Here's how the part is built. I have some questions about the finished solid (model axes, mm). A direction names the side the tool comes from. Round coordinates to 2 decimals unless told otherwise and drop trailing zeros. Order: outer loops, then holes, each group sorted by start corner. A loop starts at its lowest first (then second) coordinate and runs counter-clockwise, first axis right, second up. Notation, with made-up numbers: (50, 75) -> (72, 75) arc R32 cw to (72, 104) -> close; hole circle Ø1 at (-7, 5.25). An arc over 180 degrees is marked (long way). One line per item, written item: value.
```python
from build123d import *

# Parameters (mm, degrees)
BOSS_EXTRUDE1_DEPTH = 40
SKETCH16_R          = 17.5
BOSS_EXTRUDE2_DEPTH = 3
SKETCH17_R          = 16.65
SKETCH17_R_2        = 15.5
BOSS_EXTRUDE3_DEPTH = 10
SKETCH18_R          = 8.5
CUT_EXTRUDE1_DEPTH  = 30
BOSS_EXTRUDE4_DEPTH = 3
FILLET1_R           = 1
FILLET3_R           = 1
BOSS_EXTRUDE5_START = 2
BOSS_EXTRUDE5_DEPTH = 2
CUT_EXTRUDE3_START  = -2
CUT_EXTRUDE3_DEPTH  = 2
SKETCH28_R          = 5.051145337
CUT_EXTRUDE4_DEPTH  = 10


# Read off the part's stored shape, not the designer's step: Cut-Extrude3
with BuildPart() as part:
    # Sketch13 → Boss-Extrude1 (new body)
    with BuildSketch(Plane(origin=(0, 0, 0), x_dir=(1, 0, 0), z_dir=(0, 1, 0))):
        with BuildLine():
            Line((0.65523527, 15.486144347), (0.65523527, 15.830625123))
            Line((0.65523527, 15.830625123), (1.340586782, 15.830625123))
            Line((1.340586782, 15.830625123), (1.342992881, 16.95829018))
            Line((1.342992881, 16.95829018), (0.999793375, 16.95829018))
            Line((0.999793375, 16.95829018), (0.999793375, 16.661380915))
            Line((0.999793375, 16.661380915), (0.670404475, 16.661380915))
            Line((0.670404475, 16.661380915), (0.670404475, 17.487154081))
            ThreePointArc((0.670404475, 17.487154081), (-17.5, 0), (0.670404475, -17.487154081))
            Line((0.670404475, -17.487154081), (0.670404475, -16.661380915))
            Line((0.670404475, -16.661380915), (0.999793375, -16.661380915))
            Line((0.999793375, -16.661380915), (0.999793375, -16.95829018))
            Line((0.999793375, -16.95829018), (1.342992881, -16.95829018))
            Line((1.342992881, -16.95829018), (1.340586782, -15.830625123))
            Line((1.340586782, -15.830625123), (0.65523527, -15.830625123))
            Line((0.65523527, -15.830625123), (0.65523527, -15.486144347))
            ThreePointArc((0.65523527, -15.486144347), (-15.5, 0), (0.65523527, 15.486144347))
        make_face()
    extrude(amount=BOSS_EXTRUDE1_DEPTH)

    # Sketch16 → Boss-Extrude2 (add)
    with BuildSketch(Plane(origin=(0, 40, 0), x_dir=(1, 0, 0), z_dir=(0, 1, 0))):
        with Locations(Location((0, 0, 0), (0, 0, 87.804528663))):
            Circle(SKETCH16_R)
    extrude(amount=BOSS_EXTRUDE2_DEPTH)

    # Sketch17 → Boss-Extrude3 (add)
    with BuildSketch(Plane(origin=(0, 43, 0), x_dir=(1, 0, 0), z_dir=(0, 1, 0))):
        with Locations(Location((0, 0, 0), (0, 0, 270))):
            Circle(SKETCH17_R)
        with Locations(Location((0, 0, 0), (0, 0, 270))):
            Circle(SKETCH17_R_2, mode=Mode.SUBTRACT)
    extrude(amount=BOSS_EXTRUDE3_DEPTH)

    # Sketch18 → Cut-Extrude1 (cut)
    with BuildSketch(Plane(origin=(0, 0, 0), x_dir=(0, 0, -1), z_dir=(1, 0, 0))):
        with Locations((0, 14)):
            Circle(SKETCH18_R)
    extrude(amount=-CUT_EXTRUDE1_DEPTH, mode=Mode.SUBTRACT)

    # Sketch20 → Boss-Extrude4 (add)
    with BuildSketch(Plane.XZ):
        with BuildLine():
            Line((-14.667785333, 1.448781774), (-14.667785333, -1.448781774))
            ThreePointArc((-14.667785333, -1.448781774), (-15.025977642, -1.602140032), (-15.409950004, -1.668364732))
            ThreePointArc((-15.409950004, -1.668364732), (-15.5, 0), (-15.409950004, 1.668364732))
            ThreePointArc((-15.409950004, 1.668364732), (-15.025977642, 1.602140032), (-14.667785333, 1.448781774))
        make_face()
    extrude(amount=-BOSS_EXTRUDE4_DEPTH)

    # Fillet1
    fillet1_edges = [part.edges().sort_by_distance(p)[0] for p in [
        (-15.409950004, 1.5, 1.668364732),
    ]]
    fillet(fillet1_edges, radius=FILLET1_R)

    # Fillet3
    fillet3_edges = [part.edges().sort_by_distance(p)[0] for p in [
        (-15.409950004, 1.5, -1.668364732),
    ]]
    fillet(fillet3_edges, radius=FILLET3_R)

    # Sketch25 → Boss-Extrude5 (add)
    with BuildSketch(Plane.XZ.offset(BOSS_EXTRUDE5_START)):
        with BuildLine():
            Line((-15.5, 2.560490416), (-15.5, -2.560490416))
            ThreePointArc((-15.5, -2.560490416), (-15.394165826, -2.55830223), (-15.288512543, -2.551741411))
            ThreePointArc((-15.288512543, -2.551741411), (-15.193650033, -1.934078734), (-14.750654034, -1.493328665))
            ThreePointArc((-14.750654034, -1.493328665), (-14.708906064, -1.471638632), (-14.667785333, -1.448781774))
            Line((-14.667785333, -1.448781774), (-14.667785333, 1.448781774))
            ThreePointArc((-14.667785333, 1.448781774), (-14.708906064, 1.471638632), (-14.750654034, 1.493328665))
            ThreePointArc((-14.750654034, 1.493328665), (-15.193650033, 1.934078734), (-15.288512543, 2.551741411))
            ThreePointArc((-15.288512543, 2.551741411), (-15.394165826, 2.55830223), (-15.5, 2.560490416))
        make_face()
    extrude(amount=-BOSS_EXTRUDE5_DEPTH)

    # Cut-Extrude3 outline → Cut-Extrude3 (cut)
    with BuildSketch(Plane.XZ.offset(2).offset(CUT_EXTRUDE3_START)):
        with BuildLine():
            ThreePointArc((-15.288512543, -2.551741411), (-15.28944127, -2.546076966), (-15.290337467, -2.540407283))
            Line((-15.290337467, -2.540407283), (-15.5, -1.238247673))
            Line((-15.5, -1.238247673), (-15.5, -2.560490416))
            ThreePointArc((-15.5, -2.560490416), (-15.394165826, -2.55830223), (-15.288512543, -2.551741411))
        make_face()
        with BuildLine():
            Line((-15.5, 2.560490416), (-15.5, 1.136515472))
            Line((-15.5, 1.136515472), (-15.293549726, 2.518033727))
            ThreePointArc((-15.293549726, 2.518033727), (-15.291174748, 2.53490903), (-15.288512543, 2.551741411))
            ThreePointArc((-15.288512543, 2.551741411), (-15.394165826, 2.55830223), (-15.5, 2.560490416))
        make_face()
    extrude(amount=CUT_EXTRUDE3_DEPTH, mode=Mode.SUBTRACT)

    # Sketch28 → Cut-Extrude4 (cut)
    with BuildSketch(Plane(origin=(0, 43, 0), x_dir=(1, 0, 0), z_dir=(0, 1, 0))):
        with Locations(Location((7.825464684, 0.736813233, 0), (0, 0, 270))):
            Circle(SKETCH28_R)
    extrude(amount=-CUT_EXTRUDE4_DEPTH, mode=Mode.SUBTRACT)


solid = part.part
```
Q1. I want a section at C-C on x = 0. Write out the boundary of the cut face in (y, z), then the cut area to 3 significant figures.
Answers:
outline: (0, -17.5) -> (43, -17.5) -> (43, -16.65) -> (53, -16.65) -> (53, -15.5) -> (43, -15.5) -> (43, 15.5) -> (53, 15.5) -> (53, 16.65) -> (43, 16.65) -> (43, 17.5) -> (0, 17.5) -> (0, 15.5) -> (40, 15.5) -> (40, -15.5) -> (0, -15.5) -> close
area: 288 mm2
Q2. If we mould it in two halves opening along X, with no side actions, what happens to faces 1 (the face through (-15.4, -1, 1.8)), 2 (the face through (15.368, 47.93, -2.018)), 3 (the face through (-15, 53, 5)), 4 (the face through (5, 47.93, 15.88))? For each: pulls with the +X half, pulls with the -X half, needs draft (parallel to the pull), parting line crosses it, or undercut.
Answers:
face 1: pulls with the -X half
face 2: undercut
face 3: needs draft
face 4: parting line crosses it
Q3. I want a section at B-B on z = 0. Write out the boundary of the cut face in (x, y).
Answers:
outline: (-17.5, 0) -> (-15.5, 0) -> (-15.5, -2) -> (-14.67, -2) -> (-14.67, 3) -> (-15.5, 3) -> (-15.5, 5.5) -> (-17.5, 5.5) -> close; (-17.5, 22.5) -> (-15.5, 22.5) -> (-15.5, 40) -> (2.83, 40) -> (2.83, 43) -> (-15.5, 43) -> (-15.5, 53) -> (-16.65, 53) -> (-16.65, 43) -> (-17.5, 43) -> close; (12.82, 40) -> (17.5, 40) -> (17.5, 43) -> (16.65, 43) -> (16.65, 53) -> (15.5, 53) -> (15.5, 43) -> (12.82, 43) -> close
Q4. For P1, Ø10, axis at x = 2.5, z = 6.5, coming from the -Y side; P2, Ø6, axis at x = -10, y = 43.5, coming from the +Z side; P3, Ø0.5, axis at x = 1, y = 20, coming from the -Z side, each with a flat end and sliding along its axis, tell me the tip position at first contact or that it passes through.
Answers:
P1: y = 40
P2: z = 16.02
P3: z = -16.96
Q5. I want a section at D-D on y = 49.5. Write out the boundary of the cut face in (x, z).
Answers:
outline: circle Ø33.3 at (0, 0); hole circle Ø31 at (0, 0)
Q6. I need wall thicknesses on line 1 along X through (y, z) = (47.75, 0); line 2 along Y through (x, z) = (-4.5, 11.5); line 3 along Y through (x, z) = (-16, 1.5). Which ranges of each line are inside material? Lowest first, please.
Answers:
line 1: -16.65 to -15.5, 15.5 to 16.65
line 2: 40 to 43
line 3: 0 to 5.63, 22.37 to 53
Q7. Which directions (+Z, -Z, +X, -X, +Y, -Y) give clear straight access to the entire face, cutting with the end or side of a thin tool? Please do faces 5 (the face through (-15.5, -1, 0)), 6 (the face through (-15.394, -0.986, -1.898)), 7 (the face through (-14.668, 0, 0)), 8 (the face through (16, 43, -6)).
Answers:
face 5: +Z, -Z, -X, -Y
face 6: -Z, -X, -Y
face 7: +X, -Y
face 8: +Y
Q8. I want a section at A-A on y = 7. Write out the boundary of the cut face in (x, z), then the cut area to 3 significant figures.
Answers:
outline: (-16.82, -4.82) arc R17.5 ccw to (0.67, -17.49) -> (0.67, -16.66) -> (1, -16.66) -> (1, -16.96) -> (1.34, -16.96) -> (1.34, -15.83) -> (0.66, -15.83) -> (0.66, -15.49) arc R15.5 cw to (-14.73, -4.82) -> close; (-16.82, 4.82) -> (-14.73, 4.82) arc R15.5 cw to (0.66, 15.49) -> (0.66, 15.83) -> (1.34, 15.83) -> (1.34, 16.96) -> (1, 16.96) -> (1, 16.66) -> (0.67, 16.66) -> (0.67, 17.49) arc R17.5 ccw to start
area: 88.1 mm2
